Here's how the part is built. I have some questions about the finished solid (model axes, mm). Face numbers are marked on the shaded views. A direction names the side the tool comes from. Round coordinates to 2 decimals unless told otherwise and drop trailing zeros. Write each loop counter-clockwise with the first axis right and the second up, starting at its lowest first coordinate (ties: lowest second). Pieces come first, ordered by that corner, then holes. Notation, with made-up numbers: (32.25, 38) -> (76.25, 38) arc R15 cw to (76.25, 58) -> close; hole circle Ø2 at (-25, 52.25). An arc over 180 degrees is marked (long way). Put each result on its own line as item: value. Start each with the question number.
1. Which directions (+Z, -Z, +X, -X, +Y, -Y) give clear straight access to the entire face, cutting with the end or side of a thin tool? Please do the marked faces 1 and 2.
2. For pin 1 (2 mm diameter, centred on x = 6.5, z = 5.5, fed in from -Y); pin 2 (1.8 mm diameter, centred on x = -20.6, y = -8.1, fed in from -Z); pin 3 (8 mm diameter, centred on x = 16, y = 9, fed in from -Z); pin 4 (5 mm diameter, centred on x = -1.5, y = 6, fed in from +Z), each with a flat end and sliding along its axis, tell me the tip position at first contact or that it passes through.
3. Suppose I cut it at D-D (y = -8.1). Please give me the cut outline in (x, z), then the cut area to 3 significant figures.
4. Suppose I cut it at A-A (z = -3). Please give me the cut outline in (x, y) (3 decimals).
5. Suppose I cut it at B-B (y = 14.75). Please give me the cut outline in (x, z) (3 decimals).
6. Suppose I cut it at C-C (x = 20.45). Please give me the cut outline in (y, z), then the cut area to 3 significant figures.
7. We'd pull the mould along X, two halves only. Please class the marked faces 3, 4 and 5: +X half, -X half, draft (parallel to the pull), parting line (faces both ways), or undercut.
8. I need wall thicknesses on probe 1 along Y at (x, z) = (20.45, 0.7); probe 2 along Y at (x, z) = (-20.6, 0.4); probe 3 along X at (y, z) = (1, 8.5). Which ranges of each line are inside material? Lowest first, please. Write a range as from..to.
```python
from build123d import *

# Parameters (mm, degrees)
SKETCH1_W           = 45.5
SKETCH1_H           = 20.7
BOSS_EXTRUDE1_DEPTH = 1.6
SKETCH2_R           = 8
BOSS_EXTRUDE2_DEPTH = 12.25
BOSS_EXTRUDE3_DEPTH = 3.5
SKETCH4_R           = 1.15
CUT_EXTRUDE1_DEPTH  = 3.5
SKETCH5_W           = 12.85
SKETCH5_H           = 2.6
BOSS_EXTRUDE4_DEPTH = 2.5
SKETCH6_W           = 0.75
SKETCH6_H           = 0.75
LPATTERN1_COUNT     = 5
LPATTERN1_PITCH     = 2.55


with BuildPart() as part:
    # Sketch1 → Boss-Extrude1 (new body)
    with BuildSketch(Plane.XY):
        Rectangle(SKETCH1_W, SKETCH1_H)
    extrude(amount=BOSS_EXTRUDE1_DEPTH)

    # Sketch2 → Boss-Extrude2 (add)
    with BuildSketch(Plane.XY.offset(1.6)):
        with Locations(Location((-12.56, 0.75, 0), (0, 0, 180))):
            Circle(SKETCH2_R)
        with Locations(Location((11.84, 0.75, 0), (0, 0, 180))):
            Circle(SKETCH2_R)
    extrude(amount=BOSS_EXTRUDE2_DEPTH)

    # Sketch3 → Boss-Extrude3 (add)
    with BuildSketch(Plane.XY.offset(1.6)):
        with BuildLine():
            Line((-3.2, -5.55), (3.2, -5.55))
            ThreePointArc((3.2, -5.55), (5, -7.35), (3.2, -9.15))
            Line((3.2, -9.15), (-3.2, -9.15))
            ThreePointArc((-3.2, -9.15), (-5, -7.35), (-3.2, -5.55))
        make_face()
    extrude(amount=BOSS_EXTRUDE3_DEPTH)

    # Sketch4 → Cut-Extrude1 (cut)
    with BuildSketch(Plane(origin=(0, 0, 0), x_dir=(-1, 0, 0), z_dir=(0, 0, -1))):
        with Locations((-20.45, 8.2)):
            Circle(SKETCH4_R)
        with Locations((20.6, -8.1)):
            Circle(SKETCH4_R)
    extrude(amount=-CUT_EXTRUDE1_DEPTH, mode=Mode.SUBTRACT)

    # Sketch5 → Boss-Extrude4 (add)
    with BuildSketch(Plane(origin=(0, 0, 0), x_dir=(-1, 0, 0), z_dir=(0, 0, -1))):
        with Locations((0, 8.4)):
            Rectangle(SKETCH5_W, SKETCH5_H)
    extrude(amount=BOSS_EXTRUDE4_DEPTH)

    # Sweep17: sweep along a path in Sketch7
    with BuildLine(Plane(origin=(5.14, 0, 0), x_dir=(0, -1, 0), z_dir=(1, 0, 0))) as sweep17_path:
        Line((-8.4, 2.5), (-8.4, 4))
        ThreePointArc((-8.4, 4), (-8.546446609, 4.353553391), (-8.9, 4.5))
        Line((-8.9, 4.5), (-16.3, 4.5))
    # Sketch6 → Sweep17 (sweep)
    with BuildSketch(Plane(origin=(0, 0, -2.5), x_dir=(-1, 0, 0), z_dir=(0, 0, -1))):
        with Locations((-5.14, 8.4)):
            Rectangle(SKETCH6_W, SKETCH6_H)
    sweep17 = sweep(path=sweep17_path.line)

    # LPattern1: Sweep17 ×5
    with Locations(*[(-i * LPATTERN1_PITCH, 0, 0) for i in range(1, LPATTERN1_COUNT)]):
        add(sweep17)


solid = part.part
```
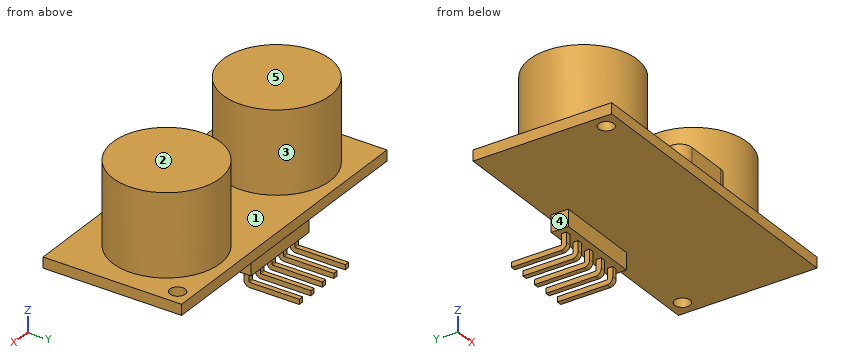
Verdict:
1. face 1: +Z
1. face 2: +Z, +X, -X, +Y, -Y
2. pin 1: stops at y = -5.97
2. pin 2: passes through
2. pin 3: stops at z = 0
2. pin 4: stops at z = 1.6
3. outline: (-22.75, 0) -> (-21.75, 0) -> (-21.75, 1.6) -> (-22.75, 1.6) -> close; (-19.45, 0) -> (22.75, 0) -> (22.75, 1.6) -> (4.84, 1.6) -> (4.84, 5.1) -> (-4.84, 5.1) -> (-4.84, 1.6) -> (-19.45, 1.6) -> close
3. area: 103 mm^2
4. outline: (-5.435, 8.025) -> (-4.685, 8.025) -> (-4.685, 8.775) -> (-5.435, 8.775) -> close; (-2.885, 8.025) -> (-2.135, 8.025) -> (-2.135, 8.775) -> (-2.885, 8.775) -> close; (-0.335, 8.025) -> (0.415, 8.025) -> (0.415, 8.775) -> (-0.335, 8.775) -> close; (2.215, 8.025) -> (2.965, 8.025) -> (2.965, 8.775) -> (2.215, 8.775) -> close; (4.765, 8.025) -> (5.515, 8.025) -> (5.515, 8.775) -> (4.765, 8.775) -> close
5. outline: (-5.435, -4.875) -> (-4.685, -4.875) -> (-4.685, -4.125) -> (-5.435, -4.125) -> close; (-2.885, -4.875) -> (-2.135, -4.875) -> (-2.135, -4.125) -> (-2.885, -4.125) -> close; (-0.335, -4.875) -> (0.415, -4.875) -> (0.415, -4.125) -> (-0.335, -4.125) -> close; (2.215, -4.875) -> (2.965, -4.875) -> (2.965, -4.125) -> (2.215, -4.125) -> close; (4.765, -4.875) -> (5.515, -4.875) -> (5.515, -4.125) -> (4.765, -4.125) -> close
6. outline: (-10.35, 0) -> (7.05, 0) -> (7.05, 1.6) -> (-10.35, 1.6) -> close; (9.35, 0) -> (10.35, 0) -> (10.35, 1.6) -> (9.35, 1.6) -> close
6. area: 29.4 mm^2
7. face 3: undercut
7. face 4: -X half
7. face 5: draft
8. probe 1: y = -10.35..7.05, 9.35..10.35
8. probe 2: y = -10.35..-9.25, -6.95..10.35
8. probe 3: x = -20.56..-4.56, 3.84..19.84
